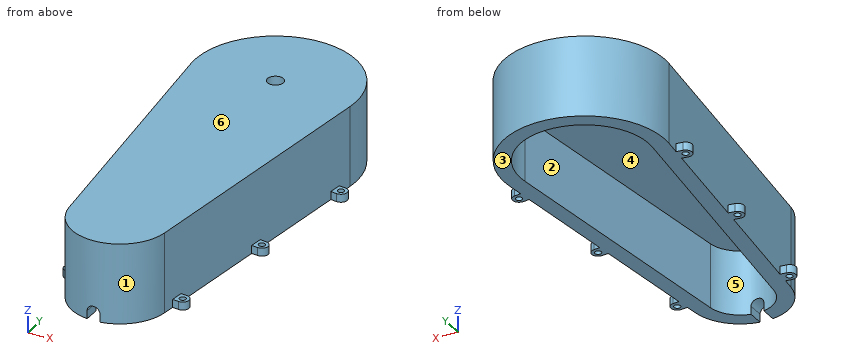
from build123d import *

# Parameters (mm, degrees)
BOSS_EXTRUDE1_DEPTH = 100
SHELL1_T            = -20
SKETCH7_R           = 10
CUT_EXTRUDE2_DEPTH  = 39
SKETCH8_R           = 4
BOSS_EXTRUDE2_DEPTH = 10
CUT_EXTRUDE3_DEPTH  = 423


with BuildPart() as part:
    # Sketch1 → Boss-Extrude1 (new body)
    with BuildSketch(Plane(origin=(0, 0, 0), x_dir=(0, 1, 0), z_dir=(0, 0, 1))):
        with BuildLine():
            Line((-356.857142857, 59.606875374), (-11.428571429, 99.34479229))
            ThreePointArc((-11.428571429, 99.34479229), (100, 0), (-11.428571429, -99.34479229))
            Line((-11.428571429, -99.34479229), (-356.857142857, -59.606875374))
            ThreePointArc((-356.857142857, -59.606875374), (-410, 0), (-356.857142857, 59.606875374))
        make_face()
    extrude(amount=BOSS_EXTRUDE1_DEPTH)

    # Shell1
    shell1_openings = [part.faces().sort_by_distance(p)[0] for p in [
        (0, -135.081480523, 0),
    ]]
    offset(amount=SHELL1_T, openings=shell1_openings, kind=Kind.INTERSECTION)

    # Sketch7 → Cut-Extrude2 (cut)
    with BuildSketch(Plane(origin=(0, 0, 80), x_dir=(1, 0, 0), z_dir=(0, 0, -1))):
        with Locations(Location((0, 0, 0), (0, 0, 180))):
            Circle(SKETCH7_R)
    extrude(amount=-CUT_EXTRUDE2_DEPTH, mode=Mode.SUBTRACT)

    # Sketch8 → Boss-Extrude2 (add)
    # profile 1 of 6: a face of its own
    with BuildSketch(Plane(origin=(0, 0, 0), x_dir=(0, 1, 0), z_dir=(0, 0, 1))):
        with BuildLine():
            Line((-342.947583383, 69.259785928), (-342.033297669, 61.312202545))
            Line((-342.033297669, 61.312202545), (-326.138130903, 63.140773973))
            Line((-326.138130903, 63.140773973), (-327.052416617, 71.088357357))
            ThreePointArc((-327.052416617, 71.088357357), (-335.914285714, 78.121655025), (-342.947583383, 69.259785928))
        make_face()
        with Locations(Location((-335, 70.174071642, 0), (0, 0, 270))):
            Circle(SKETCH8_R, mode=Mode.SUBTRACT)
    # profile 2 of 6: a face of its own
    with BuildSketch(Plane(origin=(0, 0, 0), x_dir=(0, 1, 0), z_dir=(0, 0, 1))):
        with BuildLine():
            Line((-179.552416617, 88.056677959), (-178.638130903, 80.109094575))
            Line((-178.638130903, 80.109094575), (-194.533297669, 78.280523147))
            Line((-194.533297669, 78.280523147), (-195.447583383, 86.22810653))
            ThreePointArc((-195.447583383, 86.22810653), (-188.414285714, 95.089975627), (-179.552416617, 88.056677959))
        make_face()
        with Locations(Location((-187.5, 87.142392244, 0), (0, 0, 270))):
            Circle(SKETCH8_R, mode=Mode.SUBTRACT)
    # profile 3 of 6: a face of its own
    with BuildSketch(Plane(origin=(0, 0, 0), x_dir=(0, 1, 0), z_dir=(0, 0, 1))):
        with BuildLine():
            Line((-32.052416617, 105.024998561), (-31.138130903, 97.077415177))
            Line((-31.138130903, 97.077415177), (-47.033297669, 95.248843749))
            Line((-47.033297669, 95.248843749), (-47.947583383, 103.196427132))
            ThreePointArc((-47.947583383, 103.196427132), (-40.914285714, 112.058296229), (-32.052416617, 105.024998561))
        make_face()
        with Locations(Location((-40, 104.110712846, 0), (0, 0, 270))):
            Circle(SKETCH8_R, mode=Mode.SUBTRACT)
    # profile 4 of 6: a face of its own
    with BuildSketch(Plane(origin=(0, 0, 0), x_dir=(0, 1, 0), z_dir=(0, 0, 1))):
        with BuildLine():
            Line((-47.947583383, -103.196427132), (-47.033297669, -95.248843749))
            Line((-47.033297669, -95.248843749), (-31.138130903, -97.077415177))
            Line((-31.138130903, -97.077415177), (-32.052416617, -105.024998561))
            ThreePointArc((-32.052416617, -105.024998561), (-40.914285714, -112.058296229), (-47.947583383, -103.196427132))
        make_face()
        with Locations(Location((-40, -104.110712846, 0), (0, 0, 90))):
            Circle(SKETCH8_R, mode=Mode.SUBTRACT)
    # profile 5 of 6: a face of its own
    with BuildSketch(Plane(origin=(0, 0, 0), x_dir=(0, 1, 0), z_dir=(0, 0, 1))):
        with BuildLine():
            Line((-195.447583383, -86.22810653), (-194.533297669, -78.280523147))
            Line((-194.533297669, -78.280523147), (-178.638130903, -80.109094575))
            Line((-178.638130903, -80.109094575), (-179.552416617, -88.056677959))
            ThreePointArc((-179.552416617, -88.056677959), (-188.414285714, -95.089975627), (-195.447583383, -86.22810653))
        make_face()
        with Locations(Location((-187.5, -87.142392244, 0), (0, 0, 90))):
            Circle(SKETCH8_R, mode=Mode.SUBTRACT)
    # profile 6 of 6: a face of its own
    with BuildSketch(Plane(origin=(0, 0, 0), x_dir=(0, 1, 0), z_dir=(0, 0, 1))):
        with BuildLine():
            Line((-342.033297669, -61.312202545), (-326.138130903, -63.140773973))
            Line((-326.138130903, -63.140773973), (-327.052416617, -71.088357357))
            ThreePointArc((-327.052416617, -71.088357357), (-335.914285714, -78.121655025), (-342.947583383, -69.259785928))
            Line((-342.947583383, -69.259785928), (-342.033297669, -61.312202545))
        make_face()
        with Locations(Location((-335, -70.174071642, 0), (0, 0, 90))):
            Circle(SKETCH8_R, mode=Mode.SUBTRACT)
    extrude(amount=BOSS_EXTRUDE2_DEPTH)

    # Sketch9 → Cut-Extrude3 (cut)
    with BuildSketch(Plane(origin=(0, 0, 0), x_dir=(-1, 0, 0), z_dir=(0, 1, 0))):
        with BuildLine():
            Line((0, 0), (-8, 0))
            Line((-8, 0), (-8, 10))
            ThreePointArc((-8, 10), (0, 18), (8, 10))
            Line((8, 10), (8, 0))
            Line((8, 0), (0, 0))
        make_face()
    extrude(amount=-CUT_EXTRUDE3_DEPTH, mode=Mode.SUBTRACT)


solid = part.part
Geometry: final body of the model. Coordinates: model frame, mm. Face numbers are marked on the shaded views. A direction names the side the tool comes from. Round coordinates to 2 decimals unless told otherwise and drop trailing zeros. Loops run counter-clockwise (first coordinate to the right, second up) from the corner with the lowest first, then second, coordinate; pieces in that order, holes last.
Q1. Section C-C on z = 89.5. Return loops of the section in (x, y).
Q2. Section B-B on y = 0. Return loops of the section in (x, z), plus the area to 3 significant figures.
Q3. Pull-direction query (X, two-part tool) for the marked faces 1, 2, 3 and 4; classes: released by +X, released by -X, zero draft, split by the parting line, or undercut.
Q4. Material intervals for L1, parallel to X at y = -335, z = 4; L2, parallel to Y at x = 0, z = 95.5; L3, parallel to Z at x = -11, y = -104, sorted ascending.
Q5. Access query for the marked faces 5 and 6. Directions: +Z, -Z, +X, -X, +Y, -Y. A direction counts if a zero-diameter tool reaches every point of the face in a straight line with its end or side. Return the directions, or none.
Q6. Section D-D on y = -219. Return loops of the section in (x, z), plus the area to 3 significant figures.
Q7. Pin query (flat end, axial travel): P1, Ø1, axis at x = 34, y = -322.5, coming from the -Z side; P2, Ø3, axis at y = -120, z = 23.5, coming from the +X side; P3, Ø8.5, axis at x = 86, y = -186, coming from the +Z side. Return the tip coordinate at first contact, or that it passes through.
Q8. Section A-A on x = 0. Return loops of the section in (y, z), plus the area to 3 significant figures.
Evaluation:
1. outline: (-99.34, -11.43) - (-59.61, -356.86) arc R60 ccw to (59.61, -356.86) - (99.34, -11.43) arc R100 ccw (long way) to start; hole circle Ø20 at (0, 0)
2. outline: (-100, 0) - (-80, 0) - (-80, 80) - (-10, 80) - (-10, 100) - (-100, 100) - close; (10, 80) - (80, 80) - (80, 0) - (100, 0) - (100, 100) - (10, 100) - close
2. area: 6,800 mm2
3. face 1: split by the parting line
3. face 2: undercut
3. face 3: zero draft
3. face 4: undercut
4. L1: x = -78.17 to -74.17, -66.17 to -41.99, 41.99 to 66.17, 74.17 to 78.17
4. L2: y = -410 to -10, 10 to 100
4. L3: z = 80 to 100
5. face 5: -Z
5. face 6: +Z, +X, -X, +Y, -Y
6. outline: (-75.47, 0) - (-55.33, 0) - (-55.33, 80) - (55.33, 80) - (55.33, 0) - (75.47, 0) - (75.47, 100) - (-75.47, 100) - close
6. area: 6,240 mm2
7. P1: stops at z = 80
7. P2: stops at x = 87.03
7. P3: stops at z = 10
8. outline: (-410, 18) - (-390, 18) - (-390, 80) - (-10, 80) - (-10, 100) - (-410, 100) - close; (10, 80) - (80, 80) - (80, 0) - (100, 0) - (100, 100) - (10, 100) - close
8. area: 12,600 mm2
